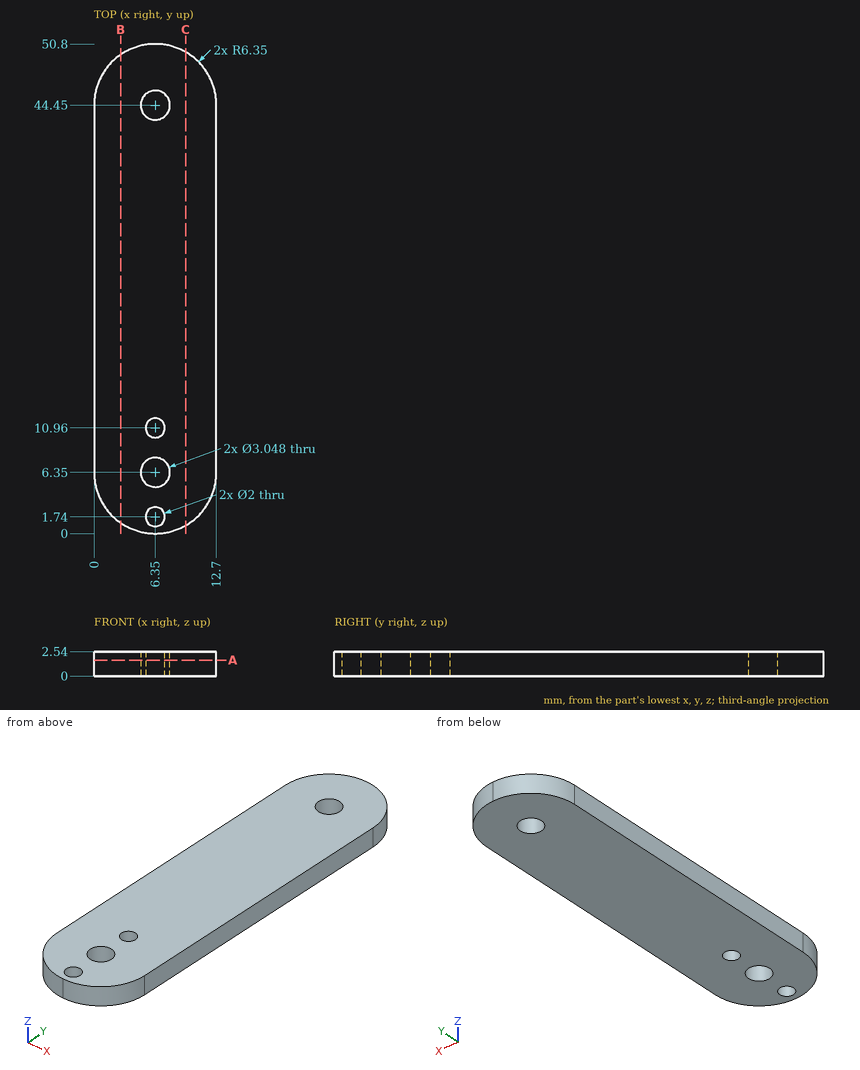
Geometry check sheet. Reference: drawing and pictorial views, mm from the part's lowest x, y, z. Give positions to 0.01 mm unless a question says otherwise; leave off trailing zeros. Order: outer loops, then holes, each group sorted by start corner. A loop starts at its lowest first (then second) coordinate and runs counter-clockwise, first axis right, second up. Notation, with made-up numbers: M -34,24 L -27,24 A18 cw -27,46 Z; hole C 32,54.25 d2. An arc over 180 degrees is marked long. Answer in a Markdown table with one row per item.
1) Cross-section at A-A, the plane z = 1.65. Enter the section's corners in (x, y), plus the area to 3 significant figures.
Filled sheet:
| item | result |
|---|---|
| outline | M 0,6.35 A6.35 ccw 12.7,6.35 L 12.7,44.45 A6.35 ccw 0,44.45 Z; hole C 6.35,6.35 d3.05; hole C 6.35,44.45 d3.05; hole C 6.35,1.74 d2; hole C 6.35,10.96 d2 |
| area | 590 mm2 |
2) Thickness scan on L1, parallel to Y at x = 6, z = 1.4; L2, parallel to X at y = 44.45, z = 2; L3, parallel to X at y = 11, z = 0.65. Record the ranges inside material, lowest first. Write a range as [from, to].
Filled sheet:
| item | result |
|---|---|
| L1 | y = [0.01, 0.8], [2.68, 4.87], [7.83, 10.02], [11.9, 42.97], [45.93, 50.79] |
| L2 | x = [0, 4.83], [7.87, 12.7] |
| L3 | x = [0, 5.35], [7.35, 12.7] |
3) Cross-section at C-C, the plane x = 9.5. Enter the section's corners in (y, z), plus the area to 3 significant figures.
Filled sheet:
| item | result |
|---|---|
| outline | M 0.84,0 L 49.96,0 L 49.96,2.54 L 0.84,2.54 Z |
| area | 125 mm2 |
4) Cross-section at B-B, the plane x = 2.75. Enter the section's corners in (y, z).
Filled sheet:
| item | result |
|---|---|
| outline | M 1.12,0 L 49.68,0 L 49.68,2.54 L 1.12,2.54 Z |
5) Gauge pin test, flat end, axial feed: P1, Ø2, axis at x = 11, y = 29.5, coming from the -Z side. Record the tip position at first contact, or that the pin passes through.
Filled sheet:
| item | result |
|---|---|
| P1 | stops at z = 0 |
